```python
from build123d import *

# Parameters (mm, degrees)
BOSS_EXTRUDE1_DEPTH = 68
CUT_EXTRUDE1_START  = -18
CUT_EXTRUDE1_DEPTH  = 18


with BuildPart() as part:
    # Sketch1 → Boss-Extrude1 (new body)
    with BuildSketch(Plane.XY):
        Polygon((0, -65.175603221), (24.260410468, -65.175603221), (24.260410468, 103.824396779), (20.214170688, 103.824396779), (20.214170688, -60.620021665), (0, -60.620021665), align=None)
    extrude(amount=BOSS_EXTRUDE1_DEPTH)

    # Sketch2 → Cut-Extrude1 (cut)
    with BuildSketch(Plane(origin=(0, 0, 0), x_dir=(-1, 0, 0), z_dir=(0, 0, -1)).offset(CUT_EXTRUDE1_START)):
        Polygon((0, -65.175603221), (0, -60.620021665), (-20.214170688, -60.620021665), (-20.214170688, 103.824396779), (-24.260410468, 103.824396779), (-24.260410468, -65.175603221), align=None)
    extrude(amount=CUT_EXTRUDE1_DEPTH, mode=Mode.SUBTRACT)


solid = part.part
```
Build history of the part. All positions in model axes, mm. A direction names the side the tool comes from. Round coordinates to 2 decimals unless told otherwise and drop trailing zeros. Write each loop counter-clockwise with the first axis right and the second up, starting at its lowest first coordinate (ties: lowest second). Pieces come first, ordered by that corner, then holes.
1) Drill centre lines: probe 1 along X at (y, z) = (42.5, 36); probe 2 along Y at (x, z) = (9.25, 27.5). Where is each one in solid material? Low to high.
2) 3-axis set-ups, long thin cutter, end or side, ignore diameter. For faces 1 (the flat face through (12, -65.176, 43)), 2 (the flat face through (20.214, 23, 43)): which of +Z, -Z, +X, -X, +Y, -Y reach the whole face in a straight line?
3) Band-saw the part on C-C, the plane x = 6.25. List the corners of the cut face in (y, z), and give its area (3 significant figures).
4) Pin check, flat tip, straight feed: pin 1 (10 mm diameter, centred on y = -6.5, z = 39, fed in from -X). Stop position of the tip, or through.
5) Band-saw the part on A-A, the plane z = 28. List the corners of the cut face in (x, y).
6) Band-saw the part on B-B, the plane y = 71. List the corners of the cut face in (x, z).
Ans:
1. probe 1: x = 20.21 to 24.26
1. probe 2: y = -65.18 to -60.62
2. face 1: +Z, -Z, +X, -X, -Y
2. face 2: +Z, -Z, -X, +Y
3. outline: (-65.18, 18) - (-60.62, 18) - (-60.62, 68) - (-65.18, 68) - close
3. area: 228 mm2
4. pin 1: stops at x = 20.21
5. outline: (0, -65.18) - (24.26, -65.18) - (24.26, 103.82) - (20.21, 103.82) - (20.21, -60.62) - (0, -60.62) - close
6. outline: (20.21, 18) - (24.26, 18) - (24.26, 68) - (20.21, 68) - close
